Could you check a few things on this model? Use its own coordinates, in mm. A direction names the side the tool comes from. Coordinates: 2 decimals unless noted, no trailing zeros. Loops run counter-clockwise (first coordinate to the right, second up) from the corner with the lowest first, then second, coordinate; pieces in that order, holes last.
from build123d import *

# Parameters (mm, degrees)
F0_R     = 32.5
F0_R_2   = 10
F1_DEPTH = 81.3
F2_DEPTH = 7.2
F3_START = 8.5
F3_DEPTH = 64.5
F4_START = 8.5
F4_DEPTH = 64.5


with BuildPart() as f1:
    # F0 (on Front) → F1 (new body)
    with BuildSketch(Plane.XZ):
        Circle(F0_R)
        with BuildLine():
            ThreePointArc((-20.255, -3.159901106), (-22.25, 0), (-20.255, 3.159901106))
            ThreePointArc((-20.255, 3.159901106), (0, 20.5), (20.255, 3.159901106))
            ThreePointArc((20.255, 3.159901106), (21.7095185419, 1.8684886941), (22.25, 0))
            ThreePointArc((22.25, 0), (21.7095185419, -1.8684886941), (20.255, -3.159901106))
            ThreePointArc((20.255, -3.159901106), (0, -20.5), (-20.255, -3.159901106))
        make_face(mode=Mode.SUBTRACT)
        with BuildLine():
            ThreePointArc((-18.1750002352, 3.4524448251), (-16.0795600384, 2.2624655603), (-15.25, 0))
            ThreePointArc((-15.25, 0), (-16.0795600384, -2.2624655603), (-18.1750002352, -3.4524448251))
            ThreePointArc((-18.1750002352, -3.4524448251), (0, -18.5000002384), (18.1750002352, -3.4524448251))
            ThreePointArc((18.1750002352, -3.4524448251), (15.25, 0), (18.1750002352, 3.4524448251))
            ThreePointArc((18.1750002352, 3.4524448251), (0, 18.5000002384), (-18.1750002352, 3.4524448251))
        make_face()
        Circle(F0_R_2, mode=Mode.SUBTRACT)
        with BuildLine():
            ThreePointArc((-20.255, 3.159901106), (-19.2374633999, 3.4658879719), (-18.1750002352, 3.4524448251))
            ThreePointArc((-18.1750002352, 3.4524448251), (0, 18.5000002384), (18.1750002352, 3.4524448251))
            ThreePointArc((18.1750002352, 3.4524448251), (19.2374633999, 3.4658879719), (20.255, 3.159901106))
            ThreePointArc((20.255, 3.159901106), (0, 20.5), (-20.255, 3.159901106))
        make_face()
        with BuildLine():
            ThreePointArc((18.1750002352, -3.4524448251), (0, -18.5000002384), (-18.1750002352, -3.4524448251))
            ThreePointArc((-18.1750002352, -3.4524448251), (-19.2374633999, -3.4658879719), (-20.255, -3.159901106))
            ThreePointArc((-20.255, -3.159901106), (0, -20.5), (20.255, -3.159901106))
            ThreePointArc((20.255, -3.159901106), (19.2374633999, -3.4658879719), (18.1750002352, -3.4524448251))
        make_face()
        with BuildLine():
            ThreePointArc((-18.1750002352, -3.4524448251), (-16.0795600384, -2.2624655603), (-15.25, 0))
            ThreePointArc((-15.25, 0), (-16.0795600384, 2.2624655603), (-18.1750002352, 3.4524448251))
            ThreePointArc((-18.1750002352, 3.4524448251), (-18.5000002384, 0), (-18.1750002352, -3.4524448251))
        make_face()
        with BuildLine():
            ThreePointArc((18.5000002384, 0), (18.4185710291, 1.7338541081), (18.1750002352, 3.4524448251))
            ThreePointArc((18.1750002352, 3.4524448251), (15.25, 0), (18.1750002352, -3.4524448251))
            ThreePointArc((18.1750002352, -3.4524448251), (18.4185710291, -1.7338541081), (18.5000002384, 0))
        make_face()
        with BuildLine():
            ThreePointArc((20.255, 3.159901106), (19.2374633999, 3.4658879719), (18.1750002352, 3.4524448251))
            ThreePointArc((18.1750002352, 3.4524448251), (18.4185710291, 1.7338541081), (18.5000002384, 0))
            ThreePointArc((18.5000002384, 0), (18.4185710291, -1.7338541081), (18.1750002352, -3.4524448251))
            ThreePointArc((18.1750002352, -3.4524448251), (19.2374633999, -3.4658879719), (20.255, -3.159901106))
            ThreePointArc((20.255, -3.159901106), (20.4386582241, -1.5846923992), (20.5, 0))
            ThreePointArc((20.5, 0), (20.4386582241, 1.5846923992), (20.255, 3.159901106))
        make_face()
        with BuildLine():
            ThreePointArc((-18.1750002352, -3.4524448251), (-18.5000002384, 0), (-18.1750002352, 3.4524448251))
            ThreePointArc((-18.1750002352, 3.4524448251), (-19.2374633999, 3.4658879719), (-20.255, 3.159901106))
            ThreePointArc((-20.255, 3.159901106), (-20.5, 0), (-20.255, -3.159901106))
            ThreePointArc((-20.255, -3.159901106), (-19.2374633999, -3.4658879719), (-18.1750002352, -3.4524448251))
        make_face()
        with BuildLine():
            ThreePointArc((22.25, 0), (21.7095185419, 1.8684886941), (20.255, 3.159901106))
            ThreePointArc((20.255, 3.159901106), (20.4386582241, 1.5846923992), (20.5, 0))
            ThreePointArc((20.5, 0), (20.4386582241, -1.5846923992), (20.255, -3.159901106))
            ThreePointArc((20.255, -3.159901106), (21.7095185419, -1.8684886941), (22.25, 0))
        make_face()
        with BuildLine():
            ThreePointArc((-20.255, -3.159901106), (-20.5, 0), (-20.255, 3.159901106))
            ThreePointArc((-20.255, 3.159901106), (-22.25, 0), (-20.255, -3.159901106))
        make_face()
    extrude(amount=F1_DEPTH)

    # F0 (on Front) → F2 (cut)
    with BuildSketch(Plane.XZ):
        with BuildLine():
            ThreePointArc((22.25, 0), (21.7095185419, 1.8684886941), (20.255, 3.159901106))
            ThreePointArc((20.255, 3.159901106), (20.4386582241, 1.5846923992), (20.5, 0))
            ThreePointArc((20.5, 0), (20.4386582241, -1.5846923992), (20.255, -3.159901106))
            ThreePointArc((20.255, -3.159901106), (21.7095185419, -1.8684886941), (22.25, 0))
        make_face()
        with BuildLine():
            ThreePointArc((20.255, 3.159901106), (19.2374633999, 3.4658879719), (18.1750002352, 3.4524448251))
            ThreePointArc((18.1750002352, 3.4524448251), (18.4185710291, 1.7338541081), (18.5000002384, 0))
            ThreePointArc((18.5000002384, 0), (18.4185710291, -1.7338541081), (18.1750002352, -3.4524448251))
            ThreePointArc((18.1750002352, -3.4524448251), (19.2374633999, -3.4658879719), (20.255, -3.159901106))
            ThreePointArc((20.255, -3.159901106), (20.4386582241, -1.5846923992), (20.5, 0))
            ThreePointArc((20.5, 0), (20.4386582241, 1.5846923992), (20.255, 3.159901106))
        make_face()
        with BuildLine():
            ThreePointArc((-20.255, -3.159901106), (-20.5, 0), (-20.255, 3.159901106))
            ThreePointArc((-20.255, 3.159901106), (-22.25, 0), (-20.255, -3.159901106))
        make_face()
        with BuildLine():
            ThreePointArc((-18.1750002352, -3.4524448251), (-18.5000002384, 0), (-18.1750002352, 3.4524448251))
            ThreePointArc((-18.1750002352, 3.4524448251), (-19.2374633999, 3.4658879719), (-20.255, 3.159901106))
            ThreePointArc((-20.255, 3.159901106), (-20.5, 0), (-20.255, -3.159901106))
            ThreePointArc((-20.255, -3.159901106), (-19.2374633999, -3.4658879719), (-18.1750002352, -3.4524448251))
        make_face()
        with BuildLine():
            ThreePointArc((-18.1750002352, -3.4524448251), (-16.0795600384, -2.2624655603), (-15.25, 0))
            ThreePointArc((-15.25, 0), (-16.0795600384, 2.2624655603), (-18.1750002352, 3.4524448251))
            ThreePointArc((-18.1750002352, 3.4524448251), (-18.5000002384, 0), (-18.1750002352, -3.4524448251))
        make_face()
        with BuildLine():
            ThreePointArc((18.5000002384, 0), (18.4185710291, 1.7338541081), (18.1750002352, 3.4524448251))
            ThreePointArc((18.1750002352, 3.4524448251), (15.25, 0), (18.1750002352, -3.4524448251))
            ThreePointArc((18.1750002352, -3.4524448251), (18.4185710291, -1.7338541081), (18.5000002384, 0))
        make_face()
    extrude(amount=F2_DEPTH, mode=Mode.SUBTRACT)

    # F0 (on Front) → F3 (cut)
    with BuildSketch(Plane.XZ.offset(F3_START)):
        Circle(F0_R)
        with BuildLine():
            ThreePointArc((-20.255, -3.159901106), (-22.25, 0), (-20.255, 3.159901106))
            ThreePointArc((-20.255, 3.159901106), (0, 20.5), (20.255, 3.159901106))
            ThreePointArc((20.255, 3.159901106), (21.7095185419, 1.8684886941), (22.25, 0))
            ThreePointArc((22.25, 0), (21.7095185419, -1.8684886941), (20.255, -3.159901106))
            ThreePointArc((20.255, -3.159901106), (0, -20.5), (-20.255, -3.159901106))
        make_face(mode=Mode.SUBTRACT)
        with BuildLine():
            ThreePointArc((-20.255, -3.159901106), (-20.5, 0), (-20.255, 3.159901106))
            ThreePointArc((-20.255, 3.159901106), (-22.25, 0), (-20.255, -3.159901106))
        make_face()
        with BuildLine():
            ThreePointArc((22.25, 0), (21.7095185419, 1.8684886941), (20.255, 3.159901106))
            ThreePointArc((20.255, 3.159901106), (20.4386582241, 1.5846923992), (20.5, 0))
            ThreePointArc((20.5, 0), (20.4386582241, -1.5846923992), (20.255, -3.159901106))
            ThreePointArc((20.255, -3.159901106), (21.7095185419, -1.8684886941), (22.25, 0))
        make_face()
    extrude(amount=F3_DEPTH, mode=Mode.SUBTRACT)

    # F0 (on Front) → F4 (cut)
    with BuildSketch(Plane.XZ.offset(F4_START)):
        with BuildLine():
            ThreePointArc((-18.1750002352, 3.4524448251), (-16.0795600384, 2.2624655603), (-15.25, 0))
            ThreePointArc((-15.25, 0), (-16.0795600384, -2.2624655603), (-18.1750002352, -3.4524448251))
            ThreePointArc((-18.1750002352, -3.4524448251), (0, -18.5000002384), (18.1750002352, -3.4524448251))
            ThreePointArc((18.1750002352, -3.4524448251), (15.25, 0), (18.1750002352, 3.4524448251))
            ThreePointArc((18.1750002352, 3.4524448251), (0, 18.5000002384), (-18.1750002352, 3.4524448251))
        make_face()
        Circle(F0_R_2, mode=Mode.SUBTRACT)
        with BuildLine():
            ThreePointArc((-18.1750002352, -3.4524448251), (-16.0795600384, -2.2624655603), (-15.25, 0))
            ThreePointArc((-15.25, 0), (-16.0795600384, 2.2624655603), (-18.1750002352, 3.4524448251))
            ThreePointArc((-18.1750002352, 3.4524448251), (-18.5000002384, 0), (-18.1750002352, -3.4524448251))
        make_face()
        with BuildLine():
            ThreePointArc((18.5000002384, 0), (18.4185710291, 1.7338541081), (18.1750002352, 3.4524448251))
            ThreePointArc((18.1750002352, 3.4524448251), (15.25, 0), (18.1750002352, -3.4524448251))
            ThreePointArc((18.1750002352, -3.4524448251), (18.4185710291, -1.7338541081), (18.5000002384, 0))
        make_face()
    extrude(amount=F4_DEPTH, mode=Mode.SUBTRACT)


solid = f1.part
(1) Which directions (+Z, -Z, +X, -X, +Y, -Y) give clear straight access to the entire face, cutting with the end or side of a thin tool? Please do faces 4 (the face through (21, -8.5, 0)), 5 (the face through (-19, -7.2, 0)), 6 (the face through (7, -81.3, 8)).
Answers:
face 4: none
face 5: +Y
face 6: +Z, -Z, +X, -X, -Y
(2) I need wall thicknesses on probe 1 along Z at (x, y) = (0, -5); probe 2 along Y at (x, z) = (-27, 3.5); probe 3 along Z at (x, y) = (-8, -43.5). Which ranges of each line are inside material? Lowest first, please.
Answers:
probe 1: z = -32.5 to -10, 10 to 32.5
probe 2: y = -81.3 to -73, -8.5 to 0
probe 3: z = -18.87 to -16.68, 16.68 to 18.87
(3) For pin 1 (8 mm diameter, centred on x = -10, y = -50, fed in from +Z); pin 2 (3.5 mm diameter, centred on x = 18, z = -0.5, fed in from +Y); pin 3 (1.5 mm diameter, centred on y = -65, z = 6, fed in from +X), each with a flat end and sliding along its axis, tell me the tip position at first contact or that it passes through.
Answers:
pin 1: stops at z = 19.6
pin 2: stops at y = -7.2
pin 3: stops at x = 19.82
(4) Imagine slicing it at B-B, the plane y = -12.5. Write out the boundary of the cut face in (x, z) (3 decimals), and give its area (3 significant figures).
Answers:
outline: circle Ø41 at (0, 0); hole circle Ø37 at (0, 0)
area: 245 mm2
(5) Imagine slicing it at A-A, the plane x = 0. Write out the boundary of the cut face in (y, z).
Answers:
outline: (-81.3, -32.5) - (-73, -32.5) - (-73, -20.5) - (-8.5, -20.5) - (-8.5, -32.5) - (0, -32.5) - (0, -10) - (-8.5, -10) - (-8.5, -18.5) - (-73, -18.5) - (-73, -10) - (-81.3, -10) - close; (-81.3, 10) - (-73, 10) - (-73, 18.5) - (-8.5, 18.5) - (-8.5, 10) - (0, 10) - (0, 32.5) - (-8.5, 32.5) - (-8.5, 20.5) - (-73, 20.5) - (-73, 32.5) - (-81.3, 32.5) - close
(6) We'd pull the mould along Y, two halves only. Please class faces 1 (the face through (19, -7.2, 0)), 2 (the face through (8, -8.5, -8)), 3 (the face through (31, -77.09, 9.76)): +Y half, -Y half, draft (parallel to the pull), parting line (faces both ways), or undercut.
Answers:
face 1: +Y half
face 2: undercut
face 3: draft
(7) Imagine slicing it at C-C, the plane z = -22.5. Write out the boundary of the cut face in (x, y), and give its area (3 significant figures).
Answers:
outline: (-23.45, -81.3) - (23.45, -81.3) - (23.45, -73) - (-23.45, -73) - close; (-23.45, -8.5) - (23.45, -8.5) - (23.45, 0) - (-23.45, 0) - close
area: 788 mm2
